from build123d import *

# Parameters (mm, degrees)
F0_R     = 1.6
F1_DEPTH = 3.175


with BuildPart() as f1:
    # F0 (on Front) → F1 (new body)
    with BuildSketch(Plane.XZ):
        with BuildLine():
            Line((26.19, 0), (3.81, 0))
            ThreePointArc((3.81, 0), (1.115923, -1.115923), (0, -3.81))
            Line((0, -3.81), (0, -56.19))
            ThreePointArc((0, -56.19), (1.115923, -58.884077), (3.81, -60))
            Line((3.81, -60), (26.19, -60))
            ThreePointArc((26.19, -60), (28.884077, -58.884077), (30, -56.19))
            Line((30, -56.19), (30, -3.81))
            ThreePointArc((30, -3.81), (28.884077, -1.115923), (26.19, 0))
        make_face()
        with Locations((5, -55)):
            Circle(F0_R, mode=Mode.SUBTRACT)
        with Locations((5, -45)):
            Circle(F0_R, mode=Mode.SUBTRACT)
        with Locations((5, -35)):
            Circle(F0_R, mode=Mode.SUBTRACT)
        with Locations((15, -55)):
            Circle(F0_R, mode=Mode.SUBTRACT)
        with Locations((25, -55)):
            Circle(F0_R, mode=Mode.SUBTRACT)
        with Locations((15, -45)):
            Circle(F0_R, mode=Mode.SUBTRACT)
        with Locations((15, -35)):
            Circle(F0_R, mode=Mode.SUBTRACT)
        with Locations((25, -45)):
            Circle(F0_R, mode=Mode.SUBTRACT)
        with Locations((25, -35)):
            Circle(F0_R, mode=Mode.SUBTRACT)
        with Locations((5, -25)):
            Circle(F0_R, mode=Mode.SUBTRACT)
        with Locations((5, -15)):
            Circle(F0_R, mode=Mode.SUBTRACT)
        with Locations((5, -5)):
            Circle(F0_R, mode=Mode.SUBTRACT)
        with Locations((15, -25)):
            Circle(F0_R, mode=Mode.SUBTRACT)
        with Locations((25, -25)):
            Circle(F0_R, mode=Mode.SUBTRACT)
        with Locations((15, -15)):
            Circle(F0_R, mode=Mode.SUBTRACT)
        with Locations((15, -5)):
            Circle(F0_R, mode=Mode.SUBTRACT)
        with Locations((25, -15)):
            Circle(F0_R, mode=Mode.SUBTRACT)
        with Locations((25, -5)):
            Circle(F0_R, mode=Mode.SUBTRACT)
    extrude(amount=F1_DEPTH)


solid = f1.part
Could you check a few things on this model? Use its own coordinates, in mm. Give positions to 0.01 mm unless a question says otherwise; leave off trailing zeros. Order: outer loops, then holes, each group sorted by start corner. A loop starts at its lowest first (then second) coordinate and runs counter-clockwise, first axis right, second up.
1. Suppose I cut it at D-D (z = -24). List the corners of the cut face in (x, y) for me (3 decimals).
2. Suppose I cut it at A-A (z = -15). List the corners of the cut face in (x, y) for me (3 decimals), plus the area to 3 significant figures.
3. Suppose I cut it at B-B (y = -0.55). Give the number of separate pieces and of enclosed holes in the cut face, plus the area to 3 significant figures.
4. I need wall thicknesses on L1, parallel to X at y = -1.4, z = -56; L2, parallel to Z at x = 3, y = -2.55; L3, parallel to Z at x = 2, y = -2. Which ranges of each line are inside material? Lowest first, please.
5. Will this pin go through, and if not, where does the flat tip stop? P1, Ø3.5, axis at x = 15, z = -25, coming from the -Y side (3 decimals).
6. We'd pull the mould along X, two halves only. Please class faces 1 (the flat face through (15, -2, -60)), 2 (the cylindrical face through (1.146, -1.565, -1.086)), 3 (the cylindrical face through (13.4, -1.57, -14.93)): pulls with the +X half, pulls with the -X half, needs draft (parallel to the pull), parting line crosses it, or undercut.
7. Suppose I cut it at C-C (x = 15). List the corners of the cut face in (y, z) for me (3 decimals).
Solved:
1. outline: (0, -3.175) - (3.751, -3.175) - (3.751, 0) - (0, 0) - close; (6.249, -3.175) - (13.751, -3.175) - (13.751, 0) - (6.249, 0) - close; (16.249, -3.175) - (23.751, -3.175) - (23.751, 0) - (16.249, 0) - close; (26.249, -3.175) - (30, -3.175) - (30, 0) - (26.249, 0) - close
2. outline: (0, -3.175) - (3.4, -3.175) - (3.4, 0) - (0, 0) - close; (6.6, -3.175) - (13.4, -3.175) - (13.4, 0) - (6.6, 0) - close; (16.6, -3.175) - (23.4, -3.175) - (23.4, 0) - (16.6, 0) - close; (26.6, -3.175) - (30, -3.175) - (30, 0) - (26.6, 0) - close
2. area: 64.8 mm2
3. separate pieces: 1
3. enclosed holes: 18
3. area: 1,640 mm2
4. L1: x = 0 to 3.75, 6.25 to 13.75, 16.25 to 23.75, 26.25 to 30
4. L2: z = -59.91 to -0.09
4. L3: z = -59.54 to -0.46
5. P1: stops at y = -3.175
6. face 1: needs draft
6. face 2: pulls with the -X half
6. face 3: undercut
7. outline: (-3.175, -60) - (0, -60) - (0, -56.6) - (-3.175, -56.6) - close; (-3.175, -53.4) - (0, -53.4) - (0, -46.6) - (-3.175, -46.6) - close; (-3.175, -43.4) - (0, -43.4) - (0, -36.6) - (-3.175, -36.6) - close; (-3.175, -33.4) - (0, -33.4) - (0, -26.6) - (-3.175, -26.6) - close; (-3.175, -23.4) - (0, -23.4) - (0, -16.6) - (-3.175, -16.6) - close; (-3.175, -13.4) - (0, -13.4) - (0, -6.6) - (-3.175, -6.6) - close; (-3.175, -3.4) - (0, -3.4) - (0, 0) - (-3.175, 0) - close
